For this review, use the dimensioned drawing (mm, ordinates from the lowest corner) and the shaded views. Give positions to 0.01 mm unless a question says otherwise; leave off trailing zeros. Write each loop counter-clockwise with the first axis right and the second up, starting at its lowest first coordinate (ties: lowest second). Pieces come first, ordered by that corner, then holes. Notation, with made-up numbers: (16, 28) -> (66, 28) arc R26 ccw to (66, 47) -> close; hole circle Ø4 at (75.25, 52). An arc over 180 degrees is marked (long way). Return JSON: item names as keys, results as strings.
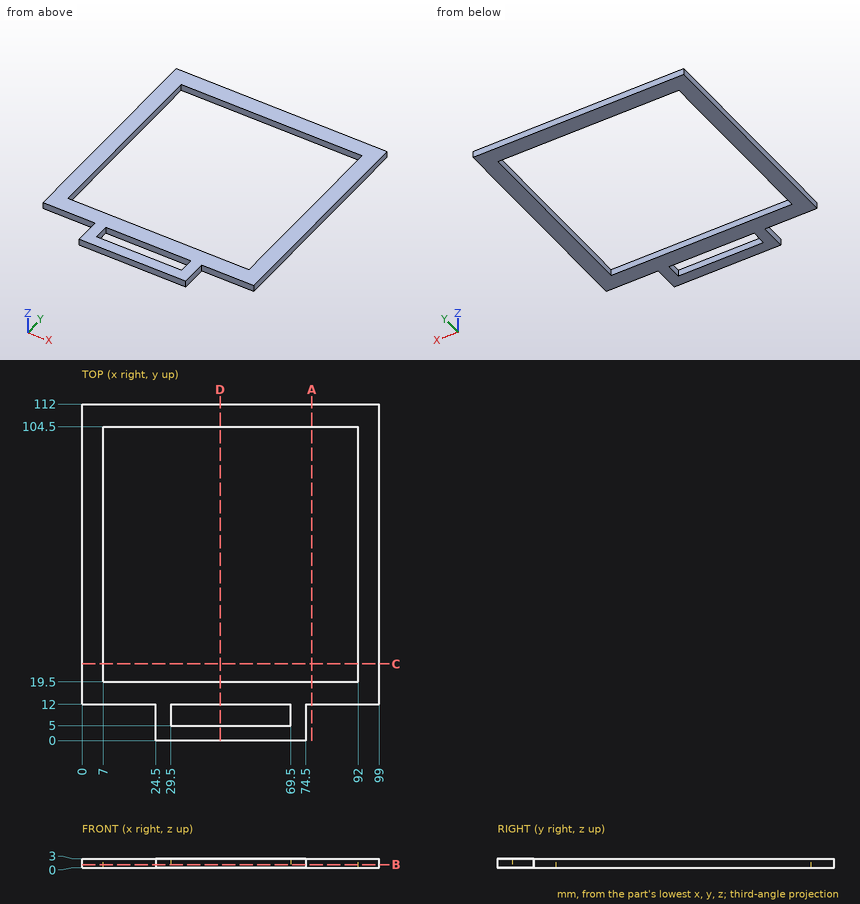
1. Add section A-A, the plane x = 76.5. State the section outline as (y, z) points.
Results found:
{"outline": "(12, 0) -> (19.5, 0) -> (19.5, 3) -> (12, 3) -> close; (104.5, 0) -> (112, 0) -> (112, 3) -> (104.5, 3) -> close"}
2. To check wall thickness, follow probe 1 along Y at (x, z) = (32.5, 1.2); probe 2 along X at (y, z) = (71, 2.5); probe 3 along Y at (x, z) = (90, 2.05). State the ranges of each line that lie inside material, in increasing order.
Results found:
{"probe 1": "y = 0 to 5, 12 to 19.5, 104.5 to 112", "probe 2": "x = 0 to 7, 92 to 99", "probe 3": "y = 12 to 19.5, 104.5 to 112"}
3. Add section D-D, the plane x = 46. State the section outline as (y, z) points.
Results found:
{"outline": "(0, 0) -> (5, 0) -> (5, 3) -> (0, 3) -> close; (12, 0) -> (19.5, 0) -> (19.5, 3) -> (12, 3) -> close; (104.5, 0) -> (112, 0) -> (112, 3) -> (104.5, 3) -> close"}
4. Add section C-C, the plane y = 25.5. State the section outline as (x, z) points, plus the area to 3 significant figures.
Results found:
{"outline": "(0, 0) -> (7, 0) -> (7, 3) -> (0, 3) -> close; (92, 0) -> (99, 0) -> (99, 3) -> (92, 3) -> close", "area": "42.0 mm²"}
5. Add section B-B, the plane z = 1. State the section outline as (x, y) points.
Results found:
{"outline": "(0, 12) -> (24.5, 12) -> (24.5, 0) -> (74.5, 0) -> (74.5, 12) -> (99, 12) -> (99, 112) -> (0, 112) -> close; hole (7, 19.5) -> (92, 19.5) -> (92, 104.5) -> (7, 104.5) -> close; hole (29.5, 5) -> (69.5, 5) -> (69.5, 12) -> (29.5, 12) -> close"}
6. For pin 1 (1.5 mm diameter, centred on y = 9, z = 2, fed in from -X); pin 2 (1.5 mm diameter, centred on x = 7, z = 2, fed in from -Y), all flat-tipped, find the tip position at first contact; note any pin that passes through.
Results found:
{"pin 1": "stops at x = 24.5", "pin 2": "stops at y = 12"}
